from build123d import *

# Parameters (mm, degrees)
BOSS_EXTRUDE1_DEPTH = 42.5
SKETCH3_R           = 42.5
BOSS_EXTRUDE2_DEPTH = 10
SKETCH4_R           = 27.5
BOSS_EXTRUDE3_DEPTH = 60
SKETCH6_W           = 90
SKETCH6_H           = 33
BOSS_EXTRUDE4_DEPTH = 92
SKETCH7_R           = 45
BOSS_EXTRUDE5_DEPTH = 22.5
SKETCH9_R           = 27.5
BOSS_EXTRUDE6_DEPTH = 35
SKETCH10_R          = 35
BOSS_EXTRUDE7_DEPTH = 7.5
SKETCH11_R          = 25
BOSS_EXTRUDE8_DEPTH = 42


with BuildPart() as part:
    # Sketch2 → Boss-Extrude1 (new, symmetric)
    with BuildSketch(Plane(origin=(0, 0, 0), x_dir=(1, 0, 0), z_dir=(0, 1, 0))):
        with BuildLine():
            Line((-45, 60), (-45, 160))
            Line((-45, 160), (45, 160))
            Line((45, 160), (45, 60))
            Line((45, 60), (45, -60))
            ThreePointArc((45, -60), (0, -75), (-45, -60))
            Line((-45, -60), (-45, 60))
        make_face()
    extrude(amount=BOSS_EXTRUDE1_DEPTH, both=True)

    # Sketch3 → Boss-Extrude2 (add)
    with BuildSketch(Plane(origin=(0, 42.5, 0), x_dir=(1, 0, 0), z_dir=(0, 1, 0))):
        with Locations((0, -7.5)):
            Circle(SKETCH3_R)
    extrude(amount=BOSS_EXTRUDE2_DEPTH)

    # Sketch4 → Boss-Extrude3 (add)
    with BuildSketch(Plane(origin=(0, 52.5, 0), x_dir=(1, 0, 0), z_dir=(0, 1, 0))):
        with Locations((0, -7.5)):
            Circle(SKETCH4_R)
    extrude(amount=BOSS_EXTRUDE3_DEPTH)

    # Sketch5 → Revolve1 (revolve)
    with BuildSketch(Plane(origin=(0, 0, 0), x_dir=(0, 0, -1), z_dir=(1, 0, 0))):
        with BuildLine():
            Line((-35, 112.5), (-7.5, 112.5))
            Line((-7.5, 112.5), (-7.5, 119.173177481))
            ThreePointArc((-7.5, 119.173177481), (-21.6490397, 117.481021512), (-35, 112.5))
        make_face()
    revolve(axis=Axis((0, 112.5, 7.5), (0, 1, 0)))

    # Sketch6 → Boss-Extrude4 (add)
    with BuildSketch(Plane(origin=(0, 42.5, 0), x_dir=(1, 0, 0), z_dir=(0, 1, 0))):
        with Locations((0, 76.5)):
            Rectangle(SKETCH6_W, SKETCH6_H)
    extrude(amount=BOSS_EXTRUDE4_DEPTH)

    # Sketch7 → Boss-Extrude5 (add)
    with BuildSketch(Plane(origin=(45, 0, 0), x_dir=(0, 0, -1), z_dir=(1, 0, 0))):
        with Locations((76.5, 39.052114436)):
            Circle(SKETCH7_R)
    extrude(amount=BOSS_EXTRUDE5_DEPTH)

    # Sketch9 → Boss-Extrude6 (add)
    with BuildSketch(Plane(origin=(67.5, 0, 0), x_dir=(0, 0, -1), z_dir=(1, 0, 0))):
        with Locations((76.5, 39.052114436)):
            Circle(SKETCH9_R)
    extrude(amount=BOSS_EXTRUDE6_DEPTH)

    # Sketch10 → Boss-Extrude7 (add)
    with BuildSketch(Plane(origin=(102.5, 0, 0), x_dir=(0, 0, -1), z_dir=(1, 0, 0))):
        with Locations((76.5, 39.052114436)):
            Circle(SKETCH10_R)
    extrude(amount=BOSS_EXTRUDE7_DEPTH)

    # Sketch11 → Boss-Extrude8 (add)
    with BuildSketch(Plane(origin=(110, 0, 0), x_dir=(0, 0, -1), z_dir=(1, 0, 0))):
        with Locations((76.5, 39.052114436)):
            Circle(SKETCH11_R)
    extrude(amount=BOSS_EXTRUDE8_DEPTH)


solid = part.part
Can you work these out from the model? Positions are in its coordinate system, mm. A direction names the side the tool comes from. Coordinates: 2 decimals unless noted, no trailing zeros. Order: outer loops, then holes, each group sorted by start corner. A loop starts at its lowest first (then second) coordinate and runs counter-clockwise, first axis right, second up. Notation, with made-up numbers: (23.25, -4) -> (36.25, -4) arc R20 ccw to (36.25, 28) -> close; hole circle Ø3 at (12, -23.75). An arc over 180 degrees is marked (long way). Use one line per item in the form item = value.
Q1. Imagine slicing it at B-B, the plane x = 0. List the corners of the cut face in (y, z) for me.
From the geometry:
outline = (-42.5, -160) -> (42.5, -160) -> (42.5, -93) -> (134.5, -93) -> (134.5, -60) -> (42.5, -60) -> (42.5, -35) -> (52.5, -35) -> (52.5, -20) -> (112.5, -20) arc R60 ccw to (112.5, 35) -> (52.5, 35) -> (52.5, 50) -> (42.5, 50) -> (42.5, 75) -> (-42.5, 75) -> close
Q2. Imagine slicing it at D-D, the plane z = 7.5. List the corners of the cut face in (x, y) for me.
From the geometry:
outline = (-45, -42.5) -> (45, -42.5) -> (45, 42.5) -> (42.5, 42.5) -> (42.5, 52.5) -> (27.5, 52.5) -> (27.5, 112.5) arc R60 ccw to (-27.5, 112.5) -> (-27.5, 52.5) -> (-42.5, 52.5) -> (-42.5, 42.5) -> (-45, 42.5) -> close
Q3. Imagine slicing it at A-A, the plane z = -76.5. List the corners of the cut face in (x, y) for me.
From the geometry:
outline = (-45, -42.5) -> (45, -42.5) -> (45, -5.95) -> (67.5, -5.95) -> (67.5, 11.55) -> (102.5, 11.55) -> (102.5, 4.05) -> (110, 4.05) -> (110, 14.05) -> (152, 14.05) -> (152, 64.05) -> (110, 64.05) -> (110, 74.05) -> (102.5, 74.05) -> (102.5, 66.55) -> (67.5, 66.55) -> (67.5, 84.05) -> (45, 84.05) -> (45, 134.5) -> (-45, 134.5) -> close
Q4. I need wall thicknesses on L1, parallel to X at y = 101, z = -85.5; L2, parallel to X at y = 47.5, z = -104.5; L3, parallel to Z at x = -6, y = 108. Which ranges of each line are inside material? Lowest first, please.
From the geometry:
L1 = -45 to 45
L2 = 45 to 67.5, 102.5 to 110
L3 = -93 to -60, -19.34 to 34.34
Q5. Imagine slicing it at C-C, the plane y = -9. List the corners of the cut face in (x, z) for me, then the cut area to 3 significant figures.
From the geometry:
outline = (-45, -160) -> (45, -160) -> (45, 60) arc R75 ccw to (-45, 60) -> close
area = 20,700 mm²
Q6. Will these pins go through, and if not, where does the flat tip stop? P1, Ø12, axis at y = 53.5, z = 47, coming from the +X side; P2, Ø10, axis at x = 52.5, z = -83.5, coming from the -Y side; P3, Ø8, axis at y = -9, z = 19, coming from the +X side.
From the geometry:
P1 = 26.05
P2 = -5.9
P3 = 45
Q7. Which directions (+Z, -Z, +X, -X, +Y, -Y) give clear straight access to the entire face, cutting with the end or side of a thin tool? Please do faces 5 (the face through (-9.21, 47.43, 48.99)), 6 (the face through (67.5, 20, -56)), 7 (the face through (45, 1, -52)).
From the geometry:
face_5 = +Y
face_6 = none
face_7 = +X, -Y
Q8. We'd pull the mould along X, two halves only. Please class faces 1 (the face through (84.755, 40.261, -49.027)), 2 (the face through (110, 47.3, -52.7)), 3 (the face through (130.71, 23.84, -56.66)), 4 (the face through (-5.961, 82.08, 34.346)): released by +X, released by -X, zero draft, split by the parting line, or undercut.
From the geometry:
face_1 = undercut
face_2 = released by +X
face_3 = zero draft
face_4 = split by the parting line
